Answer from the drawing. Dimensions are ordinates in mm from the lowest x, y and z of the part. A direction names the side the tool comes from. Give positions to 0.01 mm unless a question says otherwise; leave off trailing zeros. Write each loop counter-clockwise with the first axis right and the second up, starting at its lowest first coordinate (ties: lowest second). Pieces come first, ordered by that corner, then holes.
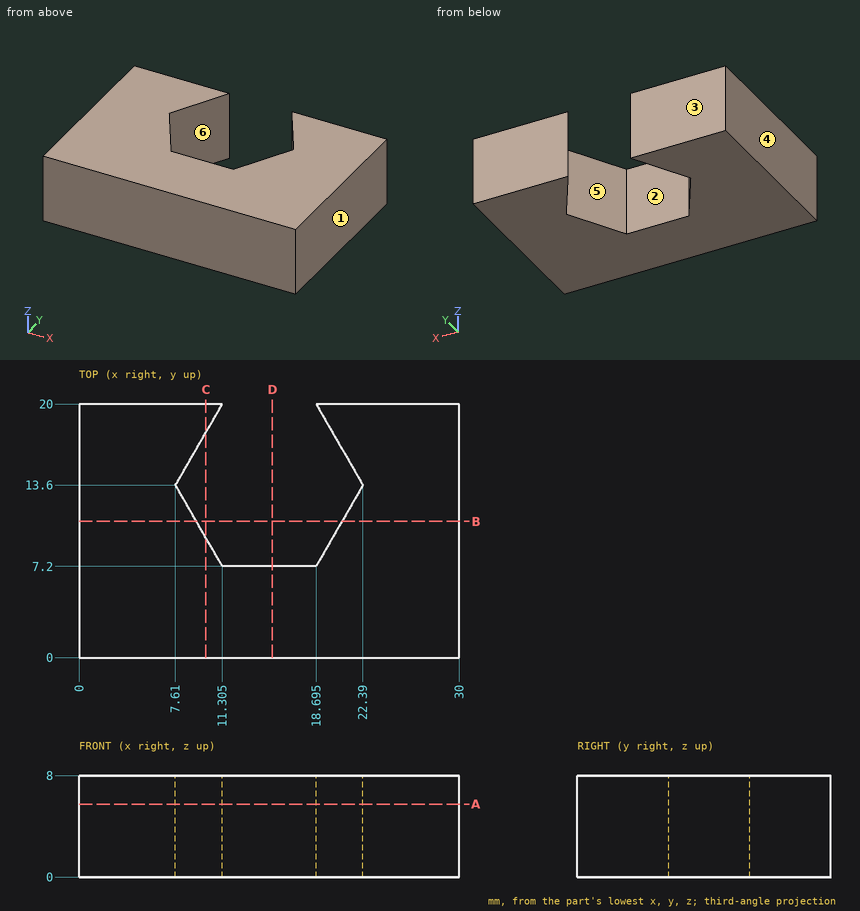
Item 1: A cutting plane is placed at C-C, the plane x = 10. Give the vertices of the cut face in (y, z).
Conclusion:
outline: (0, 0) - (9.46, 0) - (9.46, 8) - (0, 8) - close; (17.74, 0) - (20, 0) - (20, 8) - (17.74, 8) - close
Item 2: A cutting plane is placed at A-A, the plane z = 5.75. Give the vertices of the cut face in (x, y) (3 decimals), plus the area to 3 significant figures.
Conclusion:
outline: (0, 0) - (30, 0) - (30, 20) - (18.695, 20) - (22.39, 13.6) - (18.695, 7.2) - (11.305, 7.2) - (7.61, 13.6) - (11.305, 20) - (0, 20) - close
area: 458 mm2
Item 3: Consider probe 1 along X at (y, z) = (14.75, 2.5); probe 2 along X at (y, z) = (8.5, 2.5); probe 3 along Y at (x, z) = (13.5, 4.75). Determine where each line is inside the solid, lowest interval first.
Conclusion:
probe 1: x = 0 to 8.27, 21.73 to 30
probe 2: x = 0 to 10.55, 19.45 to 30
probe 3: y = 0 to 7.2
Item 4: Which of the six approach directions +Z, -Z, +X, -X, +Y, -Y give full straight-line access (tool end or side, diameter ignored) to the marked faces 1 and 2?
Conclusion:
face 1: +Z, -Z, +X, +Y, -Y
face 2: +Z, -Z, +Y
Item 5: Each of these flat-tipped pins is pushed along its axis until it touches: P1, Ø4, axis at x = 10.5, y = 11.5, coming from the +Z side; P2, Ø2, axis at x = 16, z = 3.5, coming from the +Y side. Where does it stop, or does it pass through?
Conclusion:
P1: stops at z = 8
P2: stops at y = 7.2
Item 6: A cutting plane is placed at B-B, the plane y = 10.75. Give the vertices of the cut face in (x, z).
Conclusion:
outline: (0, 0) - (9.26, 0) - (9.26, 8) - (0, 8) - close; (20.74, 0) - (30, 0) - (30, 8) - (20.74, 8) - close
Item 7: Determine the mould class of the marked faces 3, 4, 5 and 6 for opening direction X: pulls with the +X half, pulls with the -X half, needs draft (parallel to the pull), parting line crosses it, or undercut.
Conclusion:
face 3: needs draft
face 4: pulls with the -X half
face 5: undercut
face 6: undercut
Item 8: A cutting plane is placed at D-D, the plane x = 15.25. Give the vertices of the cut face in (y, z), plus the area to 3 significant figures.
Conclusion:
outline: (0, 0) - (7.2, 0) - (7.2, 8) - (0, 8) - close
area: 57.6 mm2
